from build123d import *

# Parameters (mm, degrees)
SKETCH1_R           = 19.431
SKETCH1_R_2         = 15.5625
BOSS_EXTRUDE1_DEPTH = 15
SKETCH2_R           = 19.431
BOSS_EXTRUDE2_DEPTH = 3.81
FILLET1_R           = 6.35
CHAMFER1_SIZE       = 6.35
FILLET2_R           = 6.35


with BuildPart() as part:
    # Sketch1 → Boss-Extrude1 (new body)
    with BuildSketch(Plane(origin=(0, 0, 0), x_dir=(1, 0, 0), z_dir=(0, 1, 0))):
        with Locations(Location((0, 0, 0), (0, 0, 270))):
            Circle(SKETCH1_R)
        with Locations(Location((0, 0, 0), (0, 0, 270))):
            Circle(SKETCH1_R_2, mode=Mode.SUBTRACT)
    extrude(amount=BOSS_EXTRUDE1_DEPTH)

    # Sketch2 → Boss-Extrude2 (add)
    with BuildSketch(Plane(origin=(0, 15, 0), x_dir=(1, 0, 0), z_dir=(0, 1, 0))):
        with Locations(Location((0, 0, 0), (0, 0, 270))):
            Circle(SKETCH2_R)
    extrude(amount=BOSS_EXTRUDE2_DEPTH)

    # Fillet1
    fillet1_edges = [part.edges().sort_by_distance(p)[0] for p in [
        (0, 18.81, -19.431),
    ]]
    fillet(fillet1_edges, radius=FILLET1_R)

    # Chamfer1
    # the kernel refuses this chamfer: 6.35 mm, written as the material it takes off along each edge
    with BuildSketch(Plane(origin=(0, 0, 0), x_dir=(0, 0, 1), z_dir=(-1, 0, 0))) as chamfer1_piece_1:
        Polygon((19.431, CHAMFER1_SIZE), (19.431 - CHAMFER1_SIZE, 0), (19.431, 0), align=None)
    revolve(axis=Axis((0, 0, 0), (0, 1, 0)), mode=Mode.SUBTRACT)

    # Fillet2
    fillet2_edges = [part.edges().sort_by_distance(p)[0] for p in [
        (0, 6.35, -19.431),
    ]]
    fillet(fillet2_edges, radius=FILLET2_R)


solid = part.part
Verification items for the finished model (mm, model axes). Coordinates: 2 decimals unless noted, no trailing zeros. Order: outer loops, then holes, each group sorted by start corner. A loop starts at its lowest first (then second) coordinate and runs counter-clockwise, first axis right, second up. Notation, with made-up numbers: M 38.25,-28.5 L 45.25,-28.5 A27 ccw 45.25,-11.5 Z; hole C -9.5,84.5 d7. An arc over 180 degrees is marked long. One line per item, written item: value. Start each with the question number.
Item 1: Thickness scan on probe 1 along X at (y, z) = (9, 0); probe 2 along Y at (x, z) = (-8.5, -9.5); probe 3 along Z at (x, y) = (-10, 12.25). Record the ranges inside material, lowest first.
Item 2: Sectioned sample at A-A on y = 10.5. Record the cut outline in (x, z) (1 decimal), then the cut area to 3 significant figures.
Item 3: Depth check by flat-ended pin: P1, Ø6, axis at x = -2.5, z = -11, coming from the -Y side; P2, Ø1.5, axis at x = 4.5, y = 5.5, coming from the -Z side; P3, Ø8, axis at y = 7.5, z = 14, coming from the +X side. Enter the tip coordinate at first touch or a pass-through.
Item 4: Mould release check, pull along X, two halves, no side actions. Record for faces 1 (the flat face through (0, 18.81, 0)), 2 (the flat face through (0, 15, 0)), 3 (the cylindrical face through (5.837, 10.696, 18.534)): pulls with the +X half, pulls with the -X half, needs draft (parallel to the pull), parting line crosses it, or undercut.
Item 5: Sectioned sample at B-B on y = 13.25. Record the cut outline in (x, z) (1 decimal), then the cut area to 3 significant figures.
Calculated:
1. probe 1: -19.43 to -15.56, 15.56 to 19.43
1. probe 2: 15 to 18.81
1. probe 3: -16.66 to -11.92, 11.92 to 16.66
2. outline: C 0,0 d38.9; hole C 0,0 d31.1
2. area: 425 mm^2
3. P1: y = 15
3. P2: z = -18.31
3. P3: x = 16.57
4. face 1: needs draft
4. face 2: undercut
4. face 3: parting line crosses it
5. outline: C 0,0 d38.8; hole C 0,0 d31.1
5. area: 419 mm^2
